Build history of the part. All positions in model axes, mm. Face numbers are marked on the shaded views. A direction names the side the tool comes from. Round coordinates to 2 decimals unless told otherwise and drop trailing zeros. Order: outer loops, then holes, each group sorted by start corner. A loop starts at its lowest first (then second) coordinate and runs counter-clockwise, first axis right, second up. Notation, with made-up numbers: (-11.5, 78) -> (37.5, 78) arc R11 ccw to (37.5, 83) -> close; hole circle Ø1 at (-6.5, 38). An arc over 180 degrees is marked (long way). Answer as a JSON object with one key per item and string values.
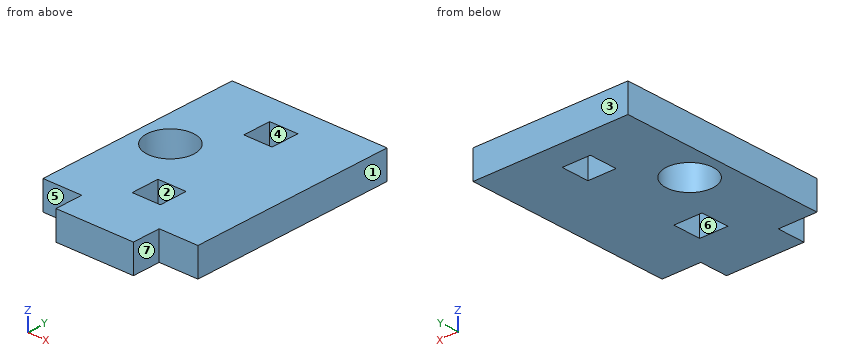
from build123d import *

# Parameters (mm, degrees)
SKETCH1_W           = 16.5
SKETCH1_H           = 22
BOSS_EXTRUDE1_DEPTH = 3
SKETCH2_W           = 8.25
SKETCH2_H           = 3
BOSS_EXTRUDE2_DEPTH = 3
SKETCH3_W           = 3
SKETCH3_H           = 3
CUT_EXTRUDE1_DEPTH  = 3
SKETCH4_R           = 2.5
CUT_EXTRUDE2_DEPTH  = 3


with BuildPart() as part:
    # Sketch1 → Boss-Extrude1 (new body)
    with BuildSketch(Plane.XY):
        Rectangle(SKETCH1_W, SKETCH1_H)
    extrude(amount=BOSS_EXTRUDE1_DEPTH)

    # Sketch2 → Boss-Extrude2 (add)
    with BuildSketch(Plane(origin=(0, -11, 0), x_dir=(-1, 0, 0), z_dir=(0, -1, 0))):
        with Locations((0, -1.5)):
            Rectangle(SKETCH2_W, SKETCH2_H)
    extrude(amount=BOSS_EXTRUDE2_DEPTH)

    # Sketch3 → Cut-Extrude1 (cut)
    with BuildSketch(Plane.XY.offset(3)):
        with Locations((0, 6.5)):
            Rectangle(SKETCH3_W, SKETCH3_H)
        with Locations((0, -6.5)):
            Rectangle(SKETCH3_W, SKETCH3_H)
    extrude(amount=-CUT_EXTRUDE1_DEPTH, mode=Mode.SUBTRACT)

    # Sketch4 → Cut-Extrude2 (cut)
    with BuildSketch(Plane.XY.offset(3)):
        with Locations((-4.75, 0)):
            Circle(SKETCH4_R)
    extrude(amount=-CUT_EXTRUDE2_DEPTH, mode=Mode.SUBTRACT)


solid = part.part
1) Flat gauge pins, fed straight in: pin 1 Ø1.5 at (x, z) = (-7, 1.5) entering from -Y; pin 2 Ø0.9 at (y, z) = (-13, 1.5) entering from -X (3 decimals). Where does each tip first touch, or does it go through?
Checked values:
{"pin 1": "stops at y = -11", "pin 2": "stops at x = -4.125"}
2) Which spindle directions (+Z, -Z, +X, -X, +Y, -Y) get a long thin tool onto all of the face, cutting with end or side? Do the marked faces 5, 6 and 7. Say none if no direction does.
Checked values:
{"face 5": "+Z, -Z, -X, -Y", "face 6": "+Z, -Z", "face 7": "+Z, -Z, +X, -Y"}
3) Pull direction Y, two halves, no side cores. Call the marked faces 1, 2, 3 and 4: pulls with the +Y half, pulls with the -Y half, needs draft (parallel to the pull), parting line crosses it, or undercut.
Checked values:
{"face 1": "needs draft", "face 2": "undercut", "face 3": "pulls with the +Y half", "face 4": "undercut"}
4) Cut at B-B, the plane z = 1.8. Give the cut face in (x, y) (3 decimals), plus the area to 3 significant figures.
Checked values:
{"outline": "(-8.25, -11) -> (-4.125, -11) -> (-4.125, -14) -> (4.125, -14) -> (4.125, -11) -> (8.25, -11) -> (8.25, 11) -> (-8.25, 11) -> close; hole circle Ø5 at (-4.75, 0); hole (-1.5, -8) -> (1.5, -8) -> (1.5, -5) -> (-1.5, -5) -> close; hole (-1.5, 5) -> (1.5, 5) -> (1.5, 8) -> (-1.5, 8) -> close", "area": "350 mm²"}
5) Cut at D-D, the plane y = -11.5. Give the cut face in (x, z) (3 decimals).
Checked values:
{"outline": "(-4.125, 0) -> (4.125, 0) -> (4.125, 3) -> (-4.125, 3) -> close"}
6) Cut at C-C, the plane x = -4.75. Give the cut face in (y, z), plus the area to 3 significant figures.
Checked values:
{"outline": "(-11, 0) -> (-2.5, 0) -> (-2.5, 3) -> (-11, 3) -> close; (2.5, 0) -> (11, 0) -> (11, 3) -> (2.5, 3) -> close", "area": "51.0 mm²"}
7) Cut at A-A, the plane y = -2. Give the cut face in (x, z).
Checked values:
{"outline": "(-8.25, 0) -> (-6.25, 0) -> (-6.25, 3) -> (-8.25, 3) -> close; (-3.25, 0) -> (8.25, 0) -> (8.25, 3) -> (-3.25, 3) -> close"}
8) Probe L1, parallel to Y at x = 0, z = 2; L2, parallel to Y at x = -4.75, z = 0.7; L3, parallel to X at y = -5.25, z = 1.45. List the from-to ranges inside material, lowest first. Write a range as from..to.
Checked values:
{"L1": "y = -14..-8, -5..5, 8..11", "L2": "y = -11..-2.5, 2.5..11", "L3": "x = -8.25..-1.5, 1.5..8.25"}
